Verification items for the finished model (mm, model axes). A direction names the side the tool comes from. Coordinates: 2 decimals unless noted, no trailing zeros. Order: outer loops, then holes, each group sorted by start corner. A loop starts at its lowest first (then second) coordinate and runs counter-clockwise, first axis right, second up. Notation, with made-up numbers: M -31.5,69.25 L -27.5,69.25 A22 cw -27.5,99.25 Z; hole C 3,59.25 d1. An arc over 180 degrees is marked long. Write item = value, one per line.
```python
from build123d import *

# Parameters (mm, degrees)
SKETCH1_W           = 200
SKETCH1_H           = 150
BOSS_EXTRUDE1_DEPTH = 280
SKETCH2_W           = 44
SKETCH2_H           = 60
SKETCH2_W_2         = 34
SKETCH2_H_2         = 72.5
CUT_EXTRUDE1_DEPTH  = 280
CUT_EXTRUDE5_DEPTH  = 200
CUT_EXTRUDE8_DEPTH  = 44
CUT_EXTRUDE9_DEPTH  = 44
SKETCH6_W           = 112
SKETCH6_H           = 52.5
CUT_EXTRUDE7_DEPTH  = 280
FILLET1_START       = -100
FILLET1_DEPTH       = 200
FILLET1_START_2     = -76
FILLET1_2_DEPTH     = 10
FILLET1_START_3     = 66
FILLET1_3_DEPTH     = 10
FILLET1_START_4     = -66
FILLET1_4_DEPTH     = 132
FILLET1_START_5     = -281
FILLET1_5_DEPTH     = 282


with BuildPart() as part:
    # Sketch1 → Boss-Extrude1 (new body)
    with BuildSketch(Plane.XY):
        Rectangle(SKETCH1_W, SKETCH1_H)
    extrude(amount=-BOSS_EXTRUDE1_DEPTH)

    # Sketch2 → Cut-Extrude1 (cut)
    with BuildSketch(Plane.XY):
        with Locations((78, -45)):
            Rectangle(SKETCH2_W, SKETCH2_H)
        with Locations((-78, -45)):
            Rectangle(SKETCH2_W, SKETCH2_H)
        with Locations((83, 38.75)):
            Rectangle(SKETCH2_W_2, SKETCH2_H_2)
        with Locations((-83, 38.75)):
            Rectangle(SKETCH2_W_2, SKETCH2_H_2)
    extrude(amount=-CUT_EXTRUDE1_DEPTH, mode=Mode.SUBTRACT)

    # Sketch3 → Cut-Extrude5 (cut)
    with BuildSketch(Plane.ZY.offset(100)):
        Polygon((-280, 2.5), (-274.399041425, 2.5), (-252, 2.5), (-218.971094498, 75), (-280, 75), align=None)
        Polygon((-236.455453487, 12.5), (-168.766953205, 12.5), (-60.438488841, 12.5), (-94.602997447, 65), (-144.84946991, 65), (-212.537970192, 65), align=None)
        Polygon((-89.179559504, 75), (-42, 2.5), (-5.600958575, 2.5), (0, 2.5), (0, 75), align=None)
    extrude(amount=-CUT_EXTRUDE5_DEPTH, mode=Mode.SUBTRACT)

    # Sketch5 → Cut-Extrude8 (cut)
    with BuildSketch(Plane.ZY.offset(100)):
        Polygon((-264.773291637, -7.125749789), (-270.374250211, -15), (-140, -15), (-140, -7.125749789), align=None)
        Polygon((-15.226708363, -7.125749789), (-140, -7.125749789), (-140, -15), (-9.625749789, -15), align=None)
    extrude(amount=-CUT_EXTRUDE8_DEPTH, mode=Mode.SUBTRACT)

    # Sketch7 → Cut-Extrude9 (cut)
    with BuildSketch(Plane(origin=(100, 0, 0), x_dir=(0, 0, -1), z_dir=(1, 0, 0))):
        Polygon((9.625749789, -15), (15.226708363, -7.125749789), (264.773291637, -7.125749789), (270.374250211, -15), align=None)
    extrude(amount=-CUT_EXTRUDE9_DEPTH, mode=Mode.SUBTRACT)

    # Sketch6 → Cut-Extrude7 (cut)
    with BuildSketch(Plane.XY):
        with Locations((0, 38.75)):
            Rectangle(SKETCH6_W, SKETCH6_H)
    extrude(amount=-CUT_EXTRUDE7_DEPTH, mode=Mode.SUBTRACT)

    # Fillet1: read off the stored shape, not the designer's step
    # Fillet1 outline → Fillet1 (cut)
    with BuildSketch(Plane.YZ.offset(FILLET1_START)):
        with BuildLine():
            Line((-75, 0), (-75, -10))
            ThreePointArc((-75, -10), (-72.071067812, -2.928932188), (-65, 0))
            Line((-65, 0), (-75, 0))
        make_face()
        with BuildLine():
            ThreePointArc((-65, -280), (-72.071067812, -277.071067812), (-75, -270))
            Line((-75, -270), (-75, -280))
            Line((-75, -280), (-65, -280))
        make_face()
        with BuildLine():
            Line((2.5, 0), (-7.5, 0))
            ThreePointArc((-7.5, 0), (-0.428932188, -2.928932188), (2.5, -10))
            Line((2.5, -10), (2.5, 0))
        make_face()
        with BuildLine():
            ThreePointArc((2.5, -270), (-0.428932188, -277.071067812), (-7.5, -280))
            Line((-7.5, -280), (2.5, -280))
            Line((2.5, -280), (2.5, -270))
        make_face()
        with BuildLine():
            Line((75, -89.179559504), (70.454316835, -86.221444616))
            ThreePointArc((70.454316835, -86.221444616), (73.790425711, -89.835564613), (75, -94.602997447))
            Line((75, -94.602997447), (75, -89.179559504))
        make_face()
        with BuildLine():
            ThreePointArc((75, -212.537970192), (73.410042611, -217.948255145), (69.145763344, -221.638115591))
            Line((69.145763344, -221.638115591), (75, -218.971094498))
            Line((75, -218.971094498), (75, -212.537970192))
        make_face()
    extrude(amount=FILLET1_DEPTH, mode=Mode.SUBTRACT)

    # Fillet1 2 outline → Fillet1 2 (add)
    with BuildSketch(Plane.YZ.offset(FILLET1_START_2)):
        with BuildLine():
            ThreePointArc((7.045683165, -44.958114888), (3.709574289, -41.343994891), (2.5, -36.576562057))
            Line((2.5, -36.576562057), (2.5, -258.433124306))
            ThreePointArc((2.5, -258.433124306), (4.089957389, -253.022839352), (8.354236656, -249.332978906))
            Line((8.354236656, -249.332978906), (69.145763344, -221.638115591))
            ThreePointArc((69.145763344, -221.638115591), (73.410042611, -217.948255145), (75, -212.537970192))
            Line((75, -212.537970192), (75, -94.602997447))
            ThreePointArc((75, -94.602997447), (73.790425711, -89.835564613), (70.454316835, -86.221444616))
            Line((70.454316835, -86.221444616), (7.045683165, -44.958114888))
        make_face()
    extrude(amount=FILLET1_2_DEPTH)

    # Fillet1 3 outline → Fillet1 3 (add)
    with BuildSketch(Plane.YZ.offset(FILLET1_START_3)):
        with BuildLine():
            ThreePointArc((7.045683165, -44.958114888), (3.709574289, -41.343994891), (2.5, -36.576562057))
            Line((2.5, -36.576562057), (2.5, -258.433124306))
            ThreePointArc((2.5, -258.433124306), (4.089957389, -253.022839352), (8.354236656, -249.332978906))
            Line((8.354236656, -249.332978906), (69.145763344, -221.638115591))
            ThreePointArc((69.145763344, -221.638115591), (73.410042611, -217.948255145), (75, -212.537970192))
            Line((75, -212.537970192), (75, -94.602997447))
            ThreePointArc((75, -94.602997447), (73.790425711, -89.835564613), (70.454316835, -86.221444616))
            Line((70.454316835, -86.221444616), (7.045683165, -44.958114888))
        make_face()
    extrude(amount=FILLET1_3_DEPTH)

    # Fillet1 4 outline → Fillet1 4 (add)
    with BuildSketch(Plane.YZ.offset(FILLET1_START_4)):
        with BuildLine():
            ThreePointArc((7.045683165, -44.958114888), (3.709574289, -41.343994891), (2.5, -36.576562057))
            Line((2.5, -36.576562057), (2.5, -42))
            Line((2.5, -42), (7.045683165, -44.958114888))
        make_face()
        with BuildLine():
            Line((2.5, -252), (2.5, -258.433124306))
            ThreePointArc((2.5, -258.433124306), (4.089957389, -253.022839352), (8.354236656, -249.332978906))
            Line((8.354236656, -249.332978906), (2.5, -252))
        make_face()
    extrude(amount=FILLET1_4_DEPTH)

    # Fillet1 5 outline → Fillet1 5 (cut)
    with BuildSketch(Plane.XY.offset(FILLET1_START_5)):
        with BuildLine():
            ThreePointArc((56, 75), (63.071067812, 72.071067812), (66, 65))
            Line((66, 65), (66, 12.5))
            ThreePointArc((66, 12.5), (68.928932188, 5.428932188), (76, 2.5))
            Line((76, 2.5), (76, 75))
            Line((76, 75), (56, 75))
        make_face()
        with BuildLine():
            ThreePointArc((-66, 65), (-63.071067812, 72.071067812), (-56, 75))
            Line((-56, 75), (-76, 75))
            Line((-76, 75), (-76, 2.5))
            ThreePointArc((-76, 2.5), (-68.928932188, 5.428932188), (-66, 12.5))
            Line((-66, 12.5), (-66, 65))
        make_face()
        with BuildLine():
            Line((100, 2.5), (90, 2.5))
            ThreePointArc((90, 2.5), (97.071067812, -0.428932188), (100, -7.5))
            Line((100, -7.5), (100, 2.5))
        make_face()
        with BuildLine():
            Line((-90, 2.5), (-100, 2.5))
            Line((-100, 2.5), (-100, -7.5))
            ThreePointArc((-100, -7.5), (-97.071067812, -0.428932188), (-90, 2.5))
        make_face()
        with BuildLine():
            Line((56, -75), (56, -65))
            ThreePointArc((56, -65), (53.071067812, -72.071067812), (46, -75))
            Line((46, -75), (56, -75))
        make_face()
        with BuildLine():
            ThreePointArc((-46, -75), (-53.071067812, -72.071067812), (-56, -65))
            Line((-56, -65), (-56, -75))
            Line((-56, -75), (-46, -75))
        make_face()
    extrude(amount=FILLET1_5_DEPTH, mode=Mode.SUBTRACT)


solid = part.part
```
Item 1: Sectioned sample at C-C, the plane z = -30.5. Enter the section's corners in (x, y).
Report:
outline = M -99.99,-7.13 L -56,-7.13 L -56,-65 A10 ccw -46,-75 L 46,-75 A10 ccw 56,-65 L 56,-7.13 L 99.99,-7.13 A10 ccw 90,2.5 L -90,2.5 A10 ccw Z
Item 2: Scan lines: L1, parallel to Y at x = -27, z = -109; L2, parallel to X at y = -26, z = -109.5; L3, parallel to Y at x = -80.5, z = -220. Record each from-to range of solid material in increasing order. Write a range as from..to.
Report:
L1 = -75..12.5, 65..75
L2 = -56..56
L3 = -7.13..2.5
Item 3: Sectioned sample at A-A, the plane x = 14. Enter the section's corners in (y, z), then the cut area to 3 significant figures.
Report:
outline = M -75,-270 A10 ccw -65,-280 L -7.5,-280 A10 ccw 2.5,-270 L 2.5,-258.43 A10 cw 8.35,-249.33 L 12.5,-247.44 L 12.5,-48.51 L 7.05,-44.96 A10 cw 2.5,-36.58 L 2.5,-10 A10 ccw -7.5,0 L -65,0 A10 ccw -75,-10 Z; M 65,-223.53 L 69.15,-221.64 A10 ccw 75,-212.54 L 75,-94.6 A10 ccw 70.45,-86.22 L 65,-82.67 Z
area = 25,000 mm^2
Item 4: Gauge pin test, flat ends, axial feed: pin 1 (5 mm diameter, centred on x = -78.5, z = -7, fed in from -Y); pin 2 (10 mm diameter, centred on x = -49, z = -98, fed in from -Y); pin 3 (22 mm diameter, centred on x = -83, z = -84.5, fed in from -Y); pin 4 (10 mm diameter, centred on x = -63, y = 43.5, fed in from -Z). Record the tip position at first contact, or that the pin passes through.
Report:
pin_1 = -15
pin_2 = -75
pin_3 = -7.13
pin_4 = -235.6
Item 5: Sectioned sample at B-B, the plane y = 18.5. Enter the section's corners in (x, z).
Report:
outline = M -66,-244.71 L -56,-244.71 L -56,-233.72 L -66,-233.72 Z; M -66,-64.34 L -56,-64.34 L -56,-52.41 L -66,-52.41 Z; M 56,-244.71 L 66,-244.71 L 66,-233.72 L 56,-233.72 Z; M 56,-64.34 L 66,-64.34 L 66,-52.41 L 56,-52.41 Z
Item 6: Sectioned sample at D-D, the plane z = -90.5. Enter the section's corners in (x, y) (1 decimal).
Report:
outline = M -100,-7.1 L -56,-7.1 L -56,-65 A10 ccw -46,-75 L 46,-75 A10 ccw 56,-65 L 56,-7.1 L 100,-7.1 A10 ccw 90,2.5 L 76,2.5 A10 cw 66,12.5 L -66,12.5 A10 cw -76,2.5 L -90,2.5 A10 ccw Z; M -66,58.7 L -56,58.7 L -56,65 L 56,65 L 56,58.7 L 66,58.7 L 66,65 A10 ccw 60.1,74.1 L -60.1,74.1 A10 ccw -66,65 Z
Item 7: Release check for a two-part mould opening along Z. For faces 5 (the flat face through (60.93, 38.38, -77.28)), 6 (the flat face through (56, 39, -230)), 7 (the flat face through (-1, -36, 0)) record: pulls with the +Z half, pulls with the -Z half, needs draft (parallel to the pull), parting line crosses it, or undercut.
Report:
face_5 = undercut
face_6 = needs draft
face_7 = pulls with the +Z half
Item 8: Tool access check on faces 1 (the flat face through (-78, -7.126, -138)), 2 (the flat face through (-66, 39, -229)), 3 (the flat face through (-61.07, 39.12, -224.33)), 4 (the flat face through (-1, 65, -152)). Record the directions out of +Z, -Z, +X, -X, +Y, -Y that give a thin tool (end or side, any length) a straight path to the whole face; none if there is none.
Report:
face_1 = -X, -Y
face_2 = +Z, -Z, -X, +Y
face_3 = +X, -X
face_4 = none
